Build history of the part. All positions in model axes, mm. Face numbers are marked on the shaded views. A direction names the side the tool comes from. Coordinates: 2 decimals unless noted, no trailing zeros. Write each loop counter-clockwise with the first axis right and the second up, starting at its lowest first coordinate (ties: lowest second). Pieces come first, ordered by that corner, then holes.
Autodesk Inventor part; units mm, degrees
ref_plane "YZ Plane" through (0, 0, 0) normal (1, 0, 0) x (0, 1, 0)
ref_plane "XZ Plane" through (0, 0, 0) normal (0, 1, 0) x (-1, 0, 0)
ref_plane "XY Plane" through (0, 0, 0) normal (0, 0, 1) x (1, 0, 0)
sketch "Sketch1" plane through (0, 0, 0) normal (0, 1, 0) x (-1, 0, 0)
  circle A0 centre (3.4811, 6.9947) radius 6.35
  line L0 (-9.2189, 19.6947) -> (16.1811, 19.6947)
  line L1 (16.1811, 19.6947) -> (16.1811, -18.4053)
  line L2 (16.1811, -18.4053) -> (-9.2189, -18.4053)
  line L3 (-9.2189, -18.4053) -> (-9.2189, 19.6947)
  line L4 (16.1811, -18.4053) -> (16.1811, -31.1053)
  line L5 (16.1811, -31.1053) -> (-9.2189, -31.1053)
  line L6 (-9.2189, -31.1053) -> (-9.2189, -18.4053)
  point P0 (0, 0)
  dimension "d0" = 12.7
  dimension "d1" = 25.4
  dimension "d2" = 38.1
  dimension "d3" = 12.7
  dimension "d4" = 12.7
  dimension "d36" = 12.7
ref_plane "Work Plane1" through (9.2189, 0, -18.4053) normal (0, 0, -1) x (-1, 0, 0)
sketch "Sketch3" plane through (9.2189, 0, -18.4053) normal (0, 0, -1) x (-1, 0, 0)
  line L0 (25.4, 0) -> (0, 0)
  line L1 (12.7, 0) -> (12.7, 50.8)
  line L2 (0, 50.8) -> (25.4, 50.8)
  circle A0 centre (12.7, 25.4) radius 1.5875
  circle A1 centre (12.7, 38.1) radius 1.5875
  point P0 (9.2189, 0)
  dimension "d23" = 3.175
  dimension "d24" = 3.175
  dimension "d25" = 25.4
  dimension "d26" = 12.7
ref_plane "Work Plane2" through (9.2189, -0.0789, -18.4053) normal (0, 0, -1) x (-1, 0, 0)
sketch "Sketch4" plane through (9.2189, -0.0789, -18.4053) normal (0, 0, -1) x (-1, 0, 0)
  line L0 (25.4, 0) -> (0, 0)
  line L1 (0, 50.8) -> (25.4, 50.8)
  circle A0 centre (12.7, 25.4) radius 1.5875
  circle A1 centre (12.7, 38.1) radius 1.5875
  line L2 (0, 50.8) -> (0, 0)
  line L3 (0, 0) -> (25.4, 0)
  line L4 (25.4, 0) -> (25.4, 50.8)
  point P0 (9.2189, 0)
  dimension "d30" = 3.175
  dimension "d31" = 3.175
  dimension "d32" = 25.4
  dimension "d29" = 12.7
extrude "Extrusion7" add sketch "Sketch1" against normal blind 12.7
extrude "Extrusion8" add sketch "Sketch4" along normal blind 12.7
properties part number "Cylinder Cutting Jig"
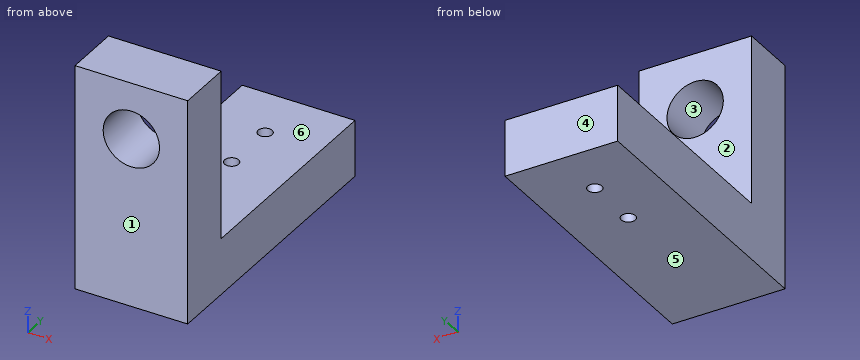
1. Saw through at B-B on x = -11.25. List the corners of the cut face in (y, z), plus the area to 3 significant figures.
Computed values:
outline: (-12.7, -31.11) - (50.72, -31.11) - (50.72, -18.41) - (0, -18.41) - (0, 19.69) - (-12.7, 19.69) - close
area: 1,290 mm2
2. Flat gauge pins, fed straight in: pin 1 (14.5 mm diameter, centred on x = -3.48, z = 6.99, fed in from -Y); pin 2 (2 mm diameter, centred on x = -2, z = -15.5, fed in from +Y); pin 3 (4 mm diameter, centred on x = -3.48, y = 25.32, fed in from +Z). Where does each tip first touch, or does it go through?
Computed values:
pin 1: stops at y = -12.7
pin 2: stops at y = 0
pin 3: stops at z = -18.41
3. Saw through at A-A on z = 3. List the corners of the cut face in (x, y), plus the area to 3 significant figures.
Computed values:
outline: (-16.18, -12.7) - (-8.42, -12.7) - (-8.42, 0) - (-16.18, 0) - close; (1.45, -12.7) - (9.22, -12.7) - (9.22, 0) - (1.45, 0) - close
area: 197 mm2
4. Saw through at D-D on z = 10. List the corners of the cut face in (x, y).
Computed values:
outline: (-16.18, -12.7) - (-9.07, -12.7) - (-9.07, 0) - (-16.18, 0) - close; (2.11, -12.7) - (9.22, -12.7) - (9.22, 0) - (2.11, 0) - close
5. 3-axis set-ups, long thin cutter, end or side, ignore diameter. For the marked faces 1 and 2: which of +Z, -Z, +X, -X, +Y, -Y reach the whole face in a straight line?
Computed values:
face 1: +Z, -Z, +X, -X, -Y
face 2: +Z, +X, -X, +Y
6. Probe line 1 along Z through (x, y) = (-5.75, 44); line 2 along Y through (x, z) = (-4, -3). List the from-to ranges inside material, lowest first.
Computed values:
line 1: z = -31.11 to -18.41
line 2: y = -12.7 to 0
7. Mould opens along Z. For the marked faces 3, 4, 5 and 6 say: +Z half, -Z half, draft (parallel to the pull), parting line (faces both ways), or undercut.
Computed values:
face 3: undercut
face 4: draft
face 5: -Z half
face 6: +Z half
8. Saw through at C-C on y = 47. List the corners of the cut face in (x, z).
Computed values:
outline: (-16.18, -31.11) - (9.22, -31.11) - (9.22, -18.41) - (-16.18, -18.41) - close
